Autodesk Inventor part; units mm, degrees
ref_plane "YZ Plane" through (0, 0, 0) normal (1, 0, 0) x (0, 1, 0)
ref_plane "XZ Plane" through (0, 0, 0) normal (0, 1, 0) x (-1, 0, 0)
ref_plane "XY Plane" through (0, 0, 0) normal (0, 0, 1) x (1, 0, 0)
ref_plane "Work Plane1" through (0, 0, 0) normal (0, 0, 1) x (1, 0, 0)
sketch "Sketch1" plane through (0, 0, 0) normal (0, 0, 1) x (1, 0, 0)
  circle A0 centre (24.1273, 54.4044) radius 16
  circle A1 centre (34.1273, 29.4044) radius 4
  circle A2 centre (49.1273, 64.4044) radius 4
  circle A3 centre (14.1273, 79.4044) radius 4
  circle A4 centre (-0.8727, 44.4044) radius 4
  circle A5 centre (-0.8727, 64.4044) radius 4
  circle A6 centre (34.1273, 79.4044) radius 4
  circle A7 centre (49.1273, 44.4044) radius 4
  circle A8 centre (14.1273, 29.4044) radius 4
  arc A9 (-5.8727, -21.5956) -> (-1.8727, -25.5956) centre (-1.8727, -21.5956) ccw
  line L0 (-1.8727, -25.5956) -> (2.1273, -25.5956)
  arc A10 (2.1273, -25.5956) -> (6.1273, -21.5956) centre (2.1273, -21.5956) ccw
  line L1 (6.1273, -21.5956) -> (6.1273, 20.4044)
  arc A11 (10.1273, 24.4044) -> (6.1273, 20.4044) centre (10.1273, 20.4044) ccw
  line L2 (10.1273, 24.4044) -> (38.1273, 24.4044)
  arc A12 (42.1273, 20.4044) -> (38.1273, 24.4044) centre (38.1273, 20.4044) ccw
  line L3 (42.1273, 20.4044) -> (42.1273, -21.5956)
  arc A13 (42.1273, -21.5956) -> (46.1273, -25.5956) centre (46.1273, -21.5956) ccw
  line L4 (46.1273, -25.5956) -> (50.1273, -25.5956)
  arc A14 (50.1273, -25.5956) -> (54.1273, -21.5956) centre (50.1273, -21.5956) ccw
  line L5 (54.1273, -21.5956) -> (54.1273, 82.4044)
  line L6 (54.1273, 82.4044) -> (52.1273, 84.4044)
  line L7 (52.1273, 84.4044) -> (-3.8727, 84.4044)
  line L8 (-3.8727, 84.4044) -> (-5.8727, 82.4044)
  line L9 (-5.8727, 82.4044) -> (-5.8727, -21.5956)
  line L10 (-5.8727, 84.4044) -> (54.1273, 84.4044)
  line L11 (54.1273, 84.4044) -> (54.1273, 24.4044)
  line L12 (54.1273, 24.4044) -> (-5.8727, 24.4044)
  line L13 (-5.8727, 24.4044) -> (-5.8727, 84.4044)
  line L14 (-5.8727, 84.4044) -> (54.1273, 24.4044) construction
  line L15 (54.1273, 84.4044) -> (-5.8727, 24.4044) construction
  circle A15 centre (24.1273, 54.4044) radius 16
  circle A16 centre (34.1273, 29.4044) radius 4
  circle A17 centre (49.1273, 64.4044) radius 4
  circle A18 centre (14.1273, 79.4044) radius 4
  circle A19 centre (-0.8727, 44.4044) radius 4
  circle A20 centre (-0.8727, 64.4044) radius 4
  circle A21 centre (34.1273, 79.4044) radius 4
  circle A22 centre (49.1273, 44.4044) radius 4
  circle A23 centre (14.1273, 29.4044) radius 4
  arc A24 (-5.8727, -21.5956) -> (-1.8727, -25.5956) centre (-1.8727, -21.5956) ccw
  line L16 (-1.8727, -25.5956) -> (2.1273, -25.5956)
  arc A25 (2.1273, -25.5956) -> (6.1273, -21.5956) centre (2.1273, -21.5956) ccw
  line L17 (6.1273, -21.5956) -> (6.1273, 20.4044)
  arc A26 (10.1273, 24.4044) -> (6.1273, 20.4044) centre (10.1273, 20.4044) ccw
  line L18 (10.1273, 24.4044) -> (38.1273, 24.4044)
  arc A27 (42.1273, 20.4044) -> (38.1273, 24.4044) centre (38.1273, 20.4044) ccw
  line L19 (42.1273, 20.4044) -> (42.1273, -21.5956)
  arc A28 (42.1273, -21.5956) -> (46.1273, -25.5956) centre (46.1273, -21.5956) ccw
  line L20 (46.1273, -25.5956) -> (50.1273, -25.5956)
  arc A29 (50.1273, -25.5956) -> (54.1273, -21.5956) centre (50.1273, -21.5956) ccw
  line L21 (54.1273, -21.5956) -> (54.1273, 82.4044)
  line L22 (54.1273, 82.4044) -> (52.1273, 84.4044)
  line L23 (52.1273, 84.4044) -> (-3.8727, 84.4044)
  line L24 (-3.8727, 84.4044) -> (-5.8727, 82.4044)
  line L25 (-5.8727, 82.4044) -> (-5.8727, -21.5956)
  circle A30 centre (-0.8727, 29.4044) radius 4
  circle A31 centre (-0.8727, 79.4044) radius 4
  circle A32 centre (49.1273, 29.4044) radius 4
  circle A33 centre (41.6273, 36.9044) radius 1.95
  circle A34 centre (41.6273, 71.9044) radius 1.95
  circle A35 centre (6.6273, 71.9044) radius 1.95
  circle A36 centre (-0.8727, 29.4044) radius 4
  circle A37 centre (-0.8727, 79.4044) radius 4
  circle A38 centre (49.1273, 29.4044) radius 4
  circle A39 centre (41.6273, 36.9044) radius 1.95
  circle A40 centre (41.6273, 71.9044) radius 1.95
  circle A41 centre (6.6273, 71.9044) radius 1.95
  circle A42 centre (49.1273, 79.4044) radius 4
  circle A43 centre (49.1273, 79.4044) radius 4
  point P0 (0, 0)
extrude "Extrusion1" add sketch "Sketch1" along normal blind 2 contours L9 L8 L7 L6 L5 L12 L2 | A33 | A34 | A35
properties part number "cellSTORM_UC2_motorized_xystage_spacer"
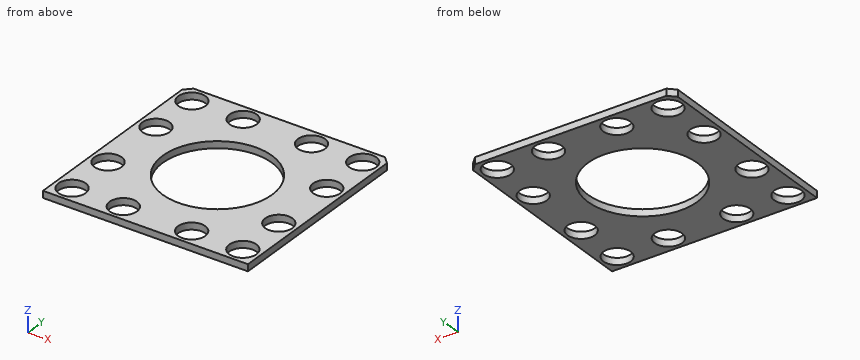
Geometry: final body of the model. Coordinates: model frame, mm. Coordinates: 2 decimals unless noted, no trailing zeros. Order: outer loops, then holes, each group sorted by start corner. A loop starts at its lowest first (then second) coordinate and runs counter-clockwise, first axis right, second up. Notation, with made-up numbers: M 59.5,47 L 91.5,47 A12 ccw 91.5,67 Z; hole C -35.75,-31 d5. An arc over 180 degrees is marked long. Answer in a Markdown table with one row per item. Add a question column.
Q1. Section query D-D on x = 23. Return the cut outline in (y, z).
Q2. Section query B-B on y = 43. Return the cut outline in (x, z).
Q3. Section query C-C on z = 1.6. Count the separate pieces of the cut face and the enclosed holes in it, and give its area (3 significant figures).
Q4. Section query A-A on x = 37. Return the cut outline in (y, z).
Q5. Line query: L1, parallel to X at y = 78, z = 0.85; L2, parallel to Y at x = 12.5, z = 0.2; L3, parallel to X at y = 80, z = 1.25. Output: solid intervals per line, ascending.
Completed:
| question | item | result |
|---|---|---|
| 1 | outline | M 24.4,0 L 38.44,0 L 38.44,2 L 24.4,2 Z; M 70.36,0 L 84.4,0 L 84.4,2 L 70.36,2 Z |
| 2 | outline | M -5.87,0 L -4.62,0 L -4.62,2 L -5.87,2 Z; M 2.87,0 L 12.91,0 L 12.91,2 L 2.87,2 Z; M 35.35,0 L 45.38,0 L 45.38,2 L 35.35,2 Z; M 52.87,0 L 54.13,0 L 54.13,2 L 52.87,2 Z |
| 3 | separate pieces | 1 |
| 3 | enclosed holes | 13 |
| 3 | area | 2,190 mm2 |
| 4 | outline | M 24.4,0 L 26.62,0 L 26.62,2 L 24.4,2 Z; M 32.19,0 L 44.9,0 L 44.9,2 L 32.19,2 Z; M 63.91,0 L 76.62,0 L 76.62,2 L 63.91,2 Z; M 82.19,0 L 84.4,0 L 84.4,2 L 82.19,2 Z |
| 5 | L1 | x = -5.87 to -4.62, 2.87 to 10.38, 17.87 to 30.38, 37.87 to 45.38, 52.87 to 54.13 |
| 5 | L2 | y = 24.4 to 25.75, 33.06 to 43.41, 65.4 to 75.75, 83.06 to 84.4 |
| 5 | L3 | x = -5.87 to -4.83, 3.08 to 10.17, 18.08 to 30.17, 38.08 to 45.17, 53.08 to 54.13 |
